Could you check a few things on this model? Use its own coordinates, in mm. Give positions to 0.01 mm unless a question says otherwise; leave off trailing zeros. Loops run counter-clockwise (first coordinate to the right, second up) from the corner with the lowest first, then second, coordinate; pieces in that order, holes last. Notation, with made-up numbers: (-11.75, 84) -> (22.25, 84) arc R29 ccw to (22.25, 120) -> close; hole circle Ø9 at (79.5, 8.5). An arc over 180 degrees is marked (long way). Write item = value, one per line. Start each with the question number.
1) I want a section at A-A (z = 1.2). List the corners of the cut face in (x, y) for me, and give its area (3 significant figures).
2) I need wall thicknesses on probe 1 along X at (y, z) = (-46.5, 1.9) (3 decimals); probe 2 along Y at (x, z) = (80, 2.15); probe 3 along Y at (x, z) = (15.5, 2.4). Which ranges of each line are inside material? Lowest first, please. Write a range as from..to.
3) I want a section at B-B (x = 24.5). List the corners of the cut face in (y, z) for me, and give its area (3 significant figures).
4) I'm going to push flat-ended pins straight in: pin 1 Ø0.9 at (x, z) = (46, 2) entering from +Y; pin 2 Ø1 at (x, y) = (38.5, -6) entering from -Z. Where does each tip first touch, or does it pass through?
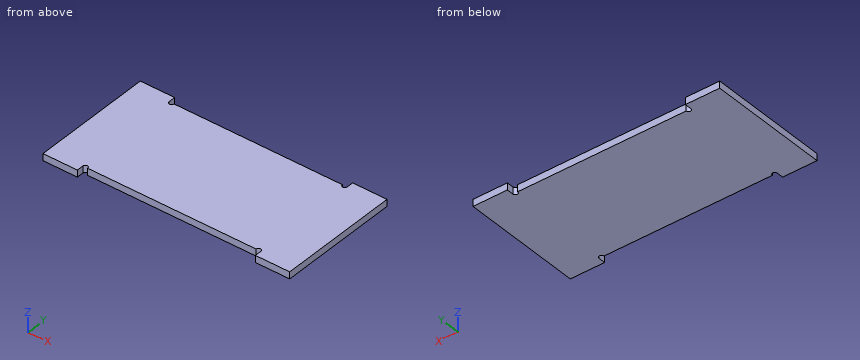
Autodesk Inventor part; units mm, degrees
ref_plane "YZ Plane" through (0, 0, 0) normal (1, 0, 0) x (0, 1, 0)
ref_plane "XZ Plane" through (0, 0, 0) normal (0, 1, 0) x (-1, 0, 0)
ref_plane "XY Plane" through (0, 0, 0) normal (0, 0, 1) x (1, 0, 0)
sketch "スケッチ1" plane through (0, 0, 0) normal (0, 0, 1) x (1, 0, 0)
  circle A0 centre (-35.9404, 22.842) radius 1.5
  circle A1 centre (5.9362, 53.5882) radius 1.5
  circle A2 centre (127.6431, 30.2622) radius 1.5
  line L0 (22.1499, 50.4807) -> (113.9448, 32.8876)
  circle A3 centre (5.9362, 53.5882) radius 4.5
  circle A4 centre (127.6431, 30.2622) radius 4.5
  circle A5 centre (-35.9404, 22.842) radius 3
  line L1 (5.0892, 49.1686) -> (11.145, 48.008)
  line L2 (11.145, 48.008) -> (22.1499, 50.4807)
  line L3 (113.9448, 32.8876) -> (122.4523, 26.6751)
  line L4 (122.4523, 26.6751) -> (126.7961, 25.8426)
  line L5 (4.4419, 57.8328) -> (15.2047, 61.622)
  line L6 (-37.785, 25.2079) -> (3.1694, 57.1371)
  line L7 (3.5126, 49.7966) -> (-34.0959, 20.4761)
  line L8 (122.0018, 41.1536) -> (130.601, 33.6535)
  circle A6 centre (80.3181, 36.2778) radius 3
  circle A7 centre (80.3181, 36.2778) radius 4.5
  line L9 (128.2106, 34.7263) -> (80.8855, 40.7419)
  circle A8 centre (80.4743, 23.124) radius 1.5
  line L10 (120.4636, 35.711) -> (121.0283, 38.6574)
  line L11 (15.1864, 58.9428) -> (14.6217, 55.9964)
  circle A9 centre (66.9779, 42.9073) radius 1.5
  circle A10 centre (66.9779, 42.9073) radius 3
  line L12 (29.9182, 56.1193) -> (29.3535, 53.1729)
  arc A11 (17.2488, 58.5475) -> (15.1864, 58.9428) centre (16.2176, 58.7451) ccw
  arc A12 (29.9182, 56.1193) -> (27.8558, 56.5146) centre (28.887, 56.3169) ccw
  arc A13 (27.2911, 53.5682) -> (29.3535, 53.1729) centre (28.3223, 53.3705) ccw
  arc A14 (14.6217, 55.9964) -> (16.6841, 55.6011) centre (15.6529, 55.7987) ccw
  line L13 (17.2488, 58.5475) -> (27.8558, 56.5146)
  line L14 (16.6841, 55.6011) -> (27.2911, 53.5682)
  arc A15 (31.8825, 55.7428) -> (27.0019, 58.7146) centre (28.887, 56.3169) ccw
  line L15 (27.0019, 58.7146) -> (18.8556, 60.2759)
  arc A16 (18.8556, 60.2759) -> (15.2047, 61.622) centre (16.2176, 58.7451) ccw
  line L16 (106.2964, 41.4808) -> (105.7317, 38.5345)
  arc A17 (108.3589, 41.0856) -> (106.2964, 41.4808) centre (107.3276, 41.2832) ccw
  arc A18 (121.0283, 38.6574) -> (118.9658, 39.0527) centre (119.997, 38.855) ccw
  arc A19 (118.4011, 36.1063) -> (120.4636, 35.711) centre (119.4323, 35.9086) ccw
  arc A20 (105.7317, 38.5345) -> (107.7942, 38.1392) centre (106.7629, 38.3368) ccw
  line L17 (31.8825, 55.7428) -> (104.3322, 41.8573)
  line L18 (108.3589, 41.0856) -> (118.9658, 39.0527)
  line L19 (107.7942, 38.1392) -> (118.4011, 36.1063)
  arc A21 (122.0018, 41.1536) -> (118.1119, 41.2527) centre (119.997, 38.855) ccw
  line L20 (118.1119, 41.2527) -> (109.9656, 42.814)
  arc A22 (109.9656, 42.814) -> (104.3322, 41.8573) centre (107.3276, 41.2832) ccw
  line L21 (30.3885, 58.9717) -> (38.2584, 54.5208)
  line L22 (16.7917, 61.7406) -> (29.4611, 59.3124)
  line L23 (120.5711, 41.8505) -> (107.9017, 44.2787)
  line L24 (106.8479, 44.2952) -> (98.5267, 42.97)
  point P0 (0, 0)
  point P1 (0, 0)
  point P2 (0, 0)
  dimension "d53" = 9
  dimension "d49" = 9
  dimension "d50" = 9
  dimension "d51" = 6
  dimension "d52" = 6
  dimension "d54" = 47.7059
  dimension "d55" = 47.7059
  dimension "d56" = 3
  dimension "d57" = 3
  dimension "d58" = 8.0769
  dimension "d59" = 8.0769
  dimension "d60" = 3
  dimension "d61" = 6
  dimension "d62" = 61.9691
  dimension "d63" = 61.9691
  dimension "d64" = 15
  dimension "d65" = 2.1
  dimension "d66" = 2
  dimension "d67" = 2
  dimension "d68" = 2
  dimension "d69" = 15
  dimension "d70" = 2.1
  dimension "d71" = 7
  dimension "d72" = 2
  dimension "d73" = 2
sketch "スケッチ2" plane through (0, 0, 0) normal (0, 0, 1) x (1, 0, 0)
  line L0 (17.1, 0) -> (90.6683, 0)
  line L1 (107.7683, 0) -> (107.7683, -47)
  line L2 (90.6683, -47) -> (17.1, -47)
  line L3 (0, -47) -> (0, 0)
  line L4 (0, 0) -> (0, 3)
  line L5 (0, 3) -> (15, 3)
  line L6 (15, 3) -> (15, 0)
  line L7 (107.7683, 0) -> (107.7683, 3)
  line L8 (107.7683, 3) -> (92.7683, 3)
  line L9 (92.7683, 3) -> (92.7683, 0)
  line L10 (107.7683, -47) -> (107.7683, -50)
  line L11 (107.7683, -50) -> (92.7683, -50)
  line L12 (92.7683, -50) -> (92.7683, -47)
  line L13 (0, -47) -> (0, -50)
  line L14 (0, -50) -> (15, -50)
  line L15 (15, -50) -> (15, -47)
  arc A0 (15, 0) -> (17.1, 0) centre (16.05, 0) ccw
  arc A1 (90.6683, 0) -> (92.7683, 0) centre (91.7183, 0) ccw
  arc A2 (92.7683, -47) -> (90.6683, -47) centre (91.7183, -47) ccw
  arc A3 (17.1, -47) -> (15, -47) centre (16.05, -47) ccw
  line L16 (15.1864, 58.9428) -> (14.6217, 55.9964)
  line L17 (120.4636, 35.711) -> (121.0283, 38.6574)
  dimension "d30" = 107.7683
  dimension "d31" = 47
  dimension "d32" = 3
  dimension "d33" = 15
  dimension "d34" = 3
  dimension "d35" = 15
  dimension "d36" = 3
  dimension "d37" = 15
  dimension "d38" = 3
  dimension "d39" = 3
  dimension "d40" = 15
  dimension "d41" = 2.1
  dimension "d42" = 2.1
  dimension "d43" = 2.1
  dimension "d44" = 2.1
  dimension "d45" = 3
  dimension "d46" = 3
  dimension "d74" = 107.7683
extrude "押し出し1" add sketch "スケッチ2" along normal blind 3
equation "\"d55\" = d54"
equation "\"d59\" = d58"
equation "\"d63\" = d62"
equation "\"d30\" = d74"
properties part number "台形サスバー板" material "ポリカーボネート、クリア"
Answer list:
q1.outline = (0, -50) -> (15, -50) -> (15, -47) arc R1.05 cw to (17.1, -47) -> (90.67, -47) arc R1.05 cw to (92.77, -47) -> (92.77, -50) -> (107.77, -50) -> (107.77, 3) -> (92.77, 3) -> (92.77, 0) arc R1.05 cw to (90.67, 0) -> (17.1, 0) arc R1.05 cw to (15, 0) -> (15, 3) -> (0, 3) -> close
q1.area = 5,240 mm^2
q2.probe_1 = 0..15.127, 16.973..90.795, 92.642..107.768
q2.probe_2 = -47..0
q2.probe_3 = -46.11..-0.89
q3.outline = (-47, 0) -> (0, 0) -> (0, 3) -> (-47, 3) -> close
q3.area = 141 mm^2
q4.pin_1 = 0
q4.pin_2 = 0
